Source: CAD feature listing. Evaluate the final solid. Frame: model axes, mm. A direction names the side the tool comes from. Give positions to 0.01 mm unless a question says otherwise; leave off trailing zeros. Write each loop counter-clockwise with the first axis right and the second up, starting at its lowest first coordinate (ties: lowest second). Pieces come first, ordered by that corner, then holes. Notation, with made-up numbers: (-16, 58) - (0, 58) arc R14 ccw to (0, 71) - close; hole circle Ø6 at (30.25, 13). An arc over 180 degrees is marked (long way). One line per question, with ' | ' between items. Start each with the question number.
(1) Section A-A, the plane x = 17.25. Return loops of the section in (y, z) (3 decimals), plus the area to 3 significant figures.
(2) Access query for faces 4 (the flat face through (13, 42, -25.4)), 5 (the flat face through (22.86, 42, -13)). Directions: +Z, -Z, +X, -X, +Y, -Y. A direction counts if a zero-diameter tool reaches every point of the face in a straight line with its end or side. Return the directions, or none.
(3) Draft query along Y for faces 1 (the cylindrical face through (24.15, 7.08, -9.13)), 2 (the flat face through (13, 42, -2.54)), 3 (the flat face through (24, 0, -13)). Return one class per face: +Y half, -Y half, draft (parallel to the pull), parting line (faces both ways), or undercut.
(4) Section D-D, the plane z = -10.25. Return loops of the section in (x, y) (3 decimals).
(5) Ray query, line 1 (X direction, y = 73.5, z = -8); line 2 (Z direction, x = 16.75, y = 50); line 3 (Z direction, x = 24, y = 9). Return the intervals inside material, ascending. Write a range as [from, to].
(6) Section B-B, the plane y = 66. Return loops of the section in (x, z), plus the area to 3 significant figures.
(7) Section C-C, the plane y = 6. Return loops of the section in (x, z), plus the area to 3 significant figures.
```python
from build123d import *

# Parameters (mm, degrees)
BOSS_EXTRUDE1_DEPTH     = 85.725
SKETCH2_R               = 3.175
CUT_EXTRUDE1_DEPTH      = 1
CUT_EXTRUDE1_DEPTH_BACK = 26.4


with BuildPart() as part:
    # Sketch1 → Boss-Extrude1 (new body)
    with BuildSketch(Plane(origin=(0, 0, 0), x_dir=(1, 0, 0), z_dir=(0, 1, 0))):
        with BuildLine():
            Line((4, 0), (21.4, 0))
            ThreePointArc((21.4, 0), (24.228427125, 1.171572875), (25.4, 4))
            Line((25.4, 4), (25.4, 21.4))
            ThreePointArc((25.4, 21.4), (24.228427125, 24.228427125), (21.4, 25.4))
            Line((21.4, 25.4), (4, 25.4))
            ThreePointArc((4, 25.4), (1.171572875, 24.228427125), (0, 21.4))
            Line((0, 21.4), (0, 4))
            ThreePointArc((0, 4), (1.171572875, 1.171572875), (4, 0))
        make_face()
        with BuildLine():
            Line((20.86, 2.54), (4.54, 2.54))
            ThreePointArc((4.54, 2.54), (3.125786438, 3.125786438), (2.54, 4.54))
            Line((2.54, 4.54), (2.54, 20.86))
            ThreePointArc((2.54, 20.86), (3.125786438, 22.274213562), (4.54, 22.86))
            Line((4.54, 22.86), (20.86, 22.86))
            ThreePointArc((20.86, 22.86), (22.274213562, 22.274213562), (22.86, 20.86))
            Line((22.86, 20.86), (22.86, 4.54))
            ThreePointArc((22.86, 4.54), (22.274213562, 3.125786438), (20.86, 2.54))
        make_face(mode=Mode.SUBTRACT)
    extrude(amount=BOSS_EXTRUDE1_DEPTH)

    # Sketch2 → Cut-Extrude1 (cut, two sides)
    with BuildSketch(Plane(origin=(25.4, 0, 0), x_dir=(0, 0, -1), z_dir=(1, 0, 0))) as cut_extrude1_sk:
        with Locations((12.303125, 6.9453125)):
            Circle(SKETCH2_R)
        with Locations((12.303125, 78.7796875)):
            Circle(SKETCH2_R)
    extrude(amount=CUT_EXTRUDE1_DEPTH, mode=Mode.SUBTRACT)
    extrude(cut_extrude1_sk.sketch, amount=-CUT_EXTRUDE1_DEPTH_BACK, mode=Mode.SUBTRACT)


solid = part.part
```
Check sheet entries:
1) outline: (0, -25.4) - (85.725, -25.4) - (85.725, -22.86) - (0, -22.86) - close; (0, -2.54) - (85.725, -2.54) - (85.725, 0) - (0, 0) - close | area: 435 mm²
2) face 4: -Z, +X, -X, +Y, -Y | face 5: +Y, -Y
3) face 1: undercut | face 2: draft | face 3: -Y half
4) outline: (0, 0) - (2.54, 0) - (2.54, 4.523) - (0, 4.523) - close; (0, 9.367) - (2.54, 9.367) - (2.54, 76.358) - (0, 76.358) - close; (0, 81.202) - (2.54, 81.202) - (2.54, 85.725) - (0, 85.725) - close; (22.86, 0) - (25.4, 0) - (25.4, 4.523) - (22.86, 4.523) - close; (22.86, 9.367) - (25.4, 9.367) - (25.4, 76.358) - (22.86, 76.358) - close; (22.86, 81.202) - (25.4, 81.202) - (25.4, 85.725) - (22.86, 85.725) - close
5) line 1: [0, 2.54], [22.86, 25.4] | line 2: [-25.4, -22.86], [-2.54, 0] | line 3: [-24.44, -14.72], [-9.88, -0.96]
6) outline: (0, -21.4) arc R4 ccw to (4, -25.4) - (21.4, -25.4) arc R4 ccw to (25.4, -21.4) - (25.4, -4) arc R4 ccw to (21.4, 0) - (4, 0) arc R4 ccw to (0, -4) - close; hole (2.54, -20.86) arc R2 ccw to (4.54, -22.86) - (20.86, -22.86) arc R2 ccw to (22.86, -20.86) - (22.86, -4.54) arc R2 ccw to (20.86, -2.54) - (4.54, -2.54) arc R2 ccw to (2.54, -4.54) - close | area: 222 mm²
7) outline: (0, -21.4) arc R4 ccw to (4, -25.4) - (21.4, -25.4) arc R4 ccw to (25.4, -21.4) - (25.4, -15.33) - (22.86, -15.33) - (22.86, -20.86) arc R2 cw to (20.86, -22.86) - (4.54, -22.86) arc R2 cw to (2.54, -20.86) - (2.54, -15.33) - (0, -15.33) - close; (0, -9.27) - (2.54, -9.27) - (2.54, -4.54) arc R2 cw to (4.54, -2.54) - (20.86, -2.54) arc R2 cw to (22.86, -4.54) - (22.86, -9.27) - (25.4, -9.27) - (25.4, -4) arc R4 ccw to (21.4, 0) - (4, 0) arc R4 ccw to (0, -4) - close | area: 191 mm²
